Geometry check sheet. Reference: the model listing, model coordinates, mm. Face numbers are marked on the shaded views. Coordinates: 2 decimals unless noted, no trailing zeros. Write each loop counter-clockwise with the first axis right and the second up, starting at its lowest first coordinate (ties: lowest second). Pieces come first, ordered by that corner, then holes. Notation, with made-up numbers: (88, -21.5) -> (99, -21.5) arc R37 ccw to (99, 15.5) -> close; hole circle Ø9 at (17, 41). An arc over 180 degrees is marked (long way). Answer as CSV lines item,"result".
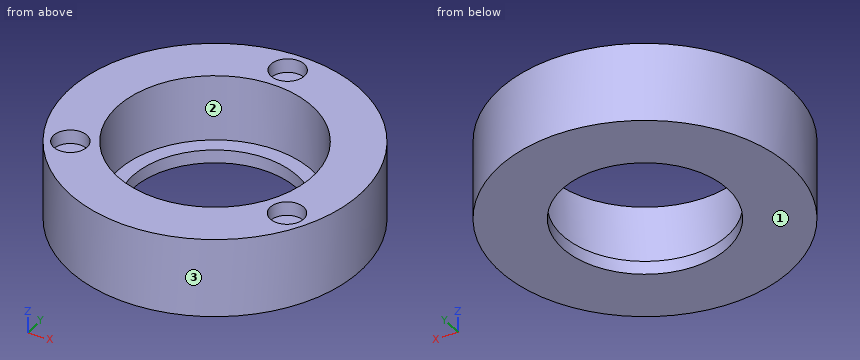
Autodesk Inventor part; units mm, degrees
ref_plane "YZ Plane" through (0, 0, 0) normal (1, 0, 0) x (0, 1, 0)
ref_plane "XZ Plane" through (0, 0, 0) normal (0, 1, 0) x (-1, 0, 0)
ref_plane "XY Plane" through (0, 0, 0) normal (0, 0, 1) x (1, 0, 0)
sketch "Skizze1" plane through (0, 0, 0) normal (0, 0, 1) x (1, 0, 0)
  circle A0 centre (0, 0) radius 22
  dimension "d0" = 44
extrude "Extrusion1" add sketch "Skizze1" along normal blind 12
sketch "Skizze2" plane through (0, 0, 12) normal (0, 0, 1) x (1, 0, 0)
  circle A0 centre (0, 18.5) radius 2.525
  point P0 (0, 0)
  dimension "d3" = 5.05
  dimension "d4" = 18.5
extrude "Extrusion2" cut sketch "Skizze2" against normal blind 2.1
pattern_circular "Runde Anordnung1" count 3 over 360 about axis through (0, 0, 0) along (0, 0, 1) of "Extrusion2"
hole "Bohrung1" at (0, 0, 12) direction (0, 0, -1) diameter 25 depth 12 counterbore diameter 29.5 counterbore depth 10
properties part number "Sensor Deckel293"
Item 1: Release check for a two-part mould opening along X. For the marked faces 1, 2 and 3 record: +X half, -X half, draft (parallel to the pull), parting line (faces both ways), or undercut.
Responses:
face 1,"draft"
face 2,"undercut"
face 3,"parting line"
Item 2: Cross-section at B-B, the plane x = 0. Record the cut outline in (y, z) (3 decimals).
Responses:
outline,"(-22, 0) -> (-12.5, 0) -> (-12.5, 2) -> (-14.75, 2) -> (-14.75, 12) -> (-22, 12) -> close; (12.5, 0) -> (22, 0) -> (22, 12) -> (21.025, 12) -> (21.025, 9.9) -> (15.975, 9.9) -> (15.975, 12) -> (14.75, 12) -> (14.75, 2) -> (12.5, 2) -> close"
Item 3: Cross-section at C-C, the plane z = 9. Record the cut outline in (x, y).
Responses:
outline,"circle Ø44 at (0, 0); hole circle Ø29.5 at (0, 0)"
Item 4: Cross-section at D-D, the plane y = 13.5. Record the cut outline in (x, z), plus the area to 3 significant figures.
Responses:
outline,"(-17.37, 0) -> (17.37, 0) -> (17.37, 12) -> (5.94, 12) -> (5.94, 2) -> (-5.94, 2) -> (-5.94, 12) -> (-17.37, 12) -> close"
area,"298 mm2"
Item 5: Cross-section at A-A, the plane y = 0. Record the cut outline in (x, z), plus the area to 3 significant figures.
Responses:
outline,"(-22, 0) -> (-12.5, 0) -> (-12.5, 2) -> (-14.75, 2) -> (-14.75, 12) -> (-22, 12) -> close; (12.5, 0) -> (22, 0) -> (22, 12) -> (14.75, 12) -> (14.75, 2) -> (12.5, 2) -> close"
area,"183 mm2"
Item 6: Depth check by flat-ended pin: pin 1 Ø4 at (y, z) = (12.5, 2) entering from -X; pin 2 Ø1.5 at (x, y) = (15.5, -10.5) entering from +Z; pin 3 Ø1 at (x, z) = (15.5, 6.5) entering from -Y. Enter the tip coordinate at first touch or a pass-through.
Responses:
pin 1,"stops at x = -19.33"
pin 2,"stops at z = 9.9"
pin 3,"stops at y = -16.09"
Item 7: Thickness scan on probe 1 along Y at (x, z) = (0, 10) (3 decimals); probe 2 along Y at (x, z) = (0, 1.1); probe 3 along Y at (x, z) = (0, 5). Record the ranges inside material, lowest first.
Responses:
probe 1,"y = -22 to -14.75, 14.75 to 15.975, 21.025 to 22"
probe 2,"y = -22 to -12.5, 12.5 to 22"
probe 3,"y = -22 to -14.75, 14.75 to 22"
